```python
from build123d import *

# Parameters (mm, degrees)
SZKIC1_W                    = 120
SZKIC1_H                    = 120
DODANIE_WYCI_GNI_CIE1_DEPTH = 67
SZKIC5_R                    = 4
WYTNIJ_WYCI_GNI_CIE1_DEPTH  = 25


with BuildPart() as part:
    # Szkic1 → Dodanie-wyciągnięcie1 (new body)
    with BuildSketch(Plane.XY):
        with Locations((60, 60)):
            Rectangle(SZKIC1_W, SZKIC1_H)
    extrude(amount=DODANIE_WYCI_GNI_CIE1_DEPTH)

    # Szkic5 → Wytnij-wyciągnięcie1 (cut)
    with BuildSketch(Plane.XY.offset(67)):
        with Locations((7, 113)):
            Circle(SZKIC5_R)
        with Locations((7, 7)):
            Circle(SZKIC5_R)
        with Locations(Location((113, 113, 0), (0, 0, 180))):
            Circle(SZKIC5_R)
        with Locations(Location((113, 7, 0), (0, 0, 180))):
            Circle(SZKIC5_R)
    extrude(amount=-WYTNIJ_WYCI_GNI_CIE1_DEPTH, mode=Mode.SUBTRACT)


solid = part.part
```
Work out the finished part from the listing and answer in its coordinate system (mm). A direction names the side the tool comes from. Round coordinates to 2 decimals unless told otherwise and drop trailing zeros. Write each loop counter-clockwise with the first axis right and the second up, starting at its lowest first coordinate (ties: lowest second). Pieces come first, ordered by that corner, then holes. Notation, with made-up numbers: (16.25, 29) -> (39.25, 29) arc R21 ccw to (39.25, 44) -> close; hole circle Ø7 at (19, 22). An arc over 180 degrees is marked (long way). Write each question's results on one line, items separated by ' | '.
Q1. Which of the six approach directions +Z, -Z, +X, -X, +Y, -Y give full straight-line access (tool end or side, diameter ignored) to faces 1 (the flat face through (59, 61, 0)), 2 (the cylindrical face through (113.521, 109.034, 54.675))?
Data:
face 1: -Z, +X, -X, +Y, -Y | face 2: +Z
Q2. A straight line is drawn through the part: line 1 along Y through (x, z) = (113, 47.5). Find the intervals that lie inside material, in ascending order. Write a range as [from, to].
Data:
line 1: [0, 3], [11, 109], [117, 120]
Q3. Determine the mould class of faces 3 (the flat face through (59, 61, 67)), 4 (the flat face through (59, 120, 33)), 5 (the flat face through (113, 113, 42)) for opening direction Y: released by +Y, released by -Y, zero draft, split by the parting line, or undercut.
Data:
face 3: zero draft | face 4: released by +Y | face 5: undercut
Q4. A flat-ended cylindrical pin translates along its axis: P1, Ø4, axis at x = 8, y = 114.5, coming from the +Z side. Find the tip coordinate at first contact, or state that the pin passes through.
Data:
P1: z = 42
Q5. Section A-A, the plane x = 7 is taken. Write down the section's boundary in (y, z), then the cut area to 3 significant figures.
Data:
outline: (0, 0) -> (120, 0) -> (120, 67) -> (117, 67) -> (117, 42) -> (109, 42) -> (109, 67) -> (11, 67) -> (11, 42) -> (3, 42) -> (3, 67) -> (0, 67) -> close | area: 7,640 mm^2
